```python
from build123d import *

# Parameters (mm, degrees)
PAD_DEPTH       = 15
FILLET_R        = 3
FILLET001_R     = 15
SKETCH001_R     = 2.75
POCKET_DEPTH    = 5.001
SKETCH002_R     = 5.1
PAD001_DEPTH    = 3
SKETCH003_R     = 4.1
POCKET001_DEPTH = 28.001
FILLET002_R     = 4


with BuildPart() as part:
    # Sketch → Pad (new body)
    with BuildSketch(Plane.XY):
        Polygon((0, 0), (0, 83), (5, 83), (5, 73), (25, 73), (25, 48), (135, 48), (135, 40), (5, 40), (5, 0), align=None)
    extrude(amount=PAD_DEPTH)

    # Fillet
    fillet_edges = [part.edges().sort_by_distance(p)[0] for p in [
        (25, 48, 7.5),
    ]]
    fillet(fillet_edges, radius=FILLET_R)

    # Fillet001
    fillet001_edges = [part.edges().sort_by_distance(p)[0] for p in [
        (5, 40, 7.5),
    ]]
    fillet(fillet001_edges, radius=FILLET001_R)

    # Sketch001 → Pocket (cut, through all)
    with BuildSketch(Plane.YZ.offset(5)):
        with Locations((7.5, 7.5)):
            Circle(SKETCH001_R)
        with Locations((78, 7.5)):
            Circle(SKETCH001_R)
    extrude(amount=-POCKET_DEPTH, mode=Mode.SUBTRACT)

    # Sketch002 → Pad001 (new body)
    with BuildSketch(Plane.YZ.offset(25)):
        with Locations((68, 7.5)):
            Circle(SKETCH002_R)
    extrude(amount=PAD001_DEPTH)

    # Sketch003 → Pocket001 (cut, through all)
    with BuildSketch(Plane.YZ.offset(28)):
        with Locations((68, 7.5)):
            Circle(SKETCH003_R)
    extrude(amount=-POCKET001_DEPTH, mode=Mode.SUBTRACT)

    # Fillet002
    fillet002_edges = [part.edges().sort_by_distance(p)[0] for p in [
        (77.5, 40, 15),
        (77.5, 40, 0),
    ]]
    fillet(fillet002_edges, radius=FILLET002_R)


solid = part.part
```
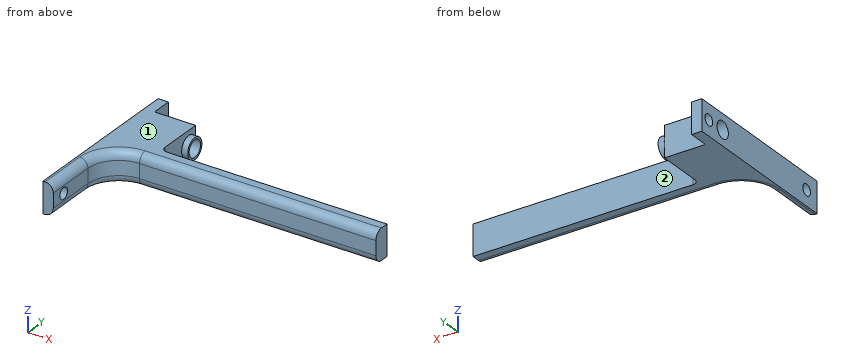
Verification items for the finished model (mm, model axes). Face numbers are marked on the shaded views. A direction names the side the tool comes from. Give positions to 0.01 mm unless a question says otherwise; leave off trailing zeros. Loops run counter-clockwise (first coordinate to the right, second up) from the corner with the lowest first, then second, coordinate; pieces in that order, holes last.
1. Section check A-A, the plane y = 7.5. Enter the section's corners in (x, z), then the cut area to 3 significant figures.
2. Set-up check for the marked faces 1 and 2: record each of +Z, -Z, +X, -X, +Y, -Y from which the full face is reachable in a straight line by a thin tool's end or side.
3. Section check C-C, the plane x = 112. Enter the section's corners in (y, z), then the cut area to 3 significant figures.
4. Section check B-B, the plane y = 78. Enter the section's corners in (x, z).
5. Section check D-D, the plane y = 68. Enter the section's corners in (x, z).
6. Thickness scan on line 1 (Z direction, x = 8, y = 68); line 2 (Z direction, x = 1.4, y = 7.5); line 3 (X direction, y = 24, z = 4). Record the ranges inside material, lowest first.
7. Go/stop test with flat-tipped pins: pin 1 Ø4 at (x, z) = (111, 7) entering from -Y; pin 2 Ø7.5 at (y, z) = (16.5, 8.5) entering from +X; pin 3 Ø7.5 at (x, z) = (17.5, 8.5) entering from +Y. Record where each tip stops, or that it passes through.
Geometry says:
1. outline: (0, 0) - (1, 0) arc R4 ccw to (5, 4) - (5, 4.75) - (0, 4.75) - close; (0, 10.25) - (5, 10.25) - (5, 11) arc R4 ccw to (1, 15) - (0, 15) - close
1. area: 40.6 mm2
2. face 1: +Z, +X, -X, +Y, -Y
2. face 2: +Z, -Z, +X, +Y
3. outline: (40, 4) arc R4 ccw to (44, 0) - (48, 0) - (48, 15) - (44, 15) arc R4 ccw to (40, 11) - close
3. area: 113 mm2
4. outline: (0, 0) - (5, 0) - (5, 4.75) - (0, 4.75) - close; (0, 10.25) - (5, 10.25) - (5, 15) - (0, 15) - close
5. outline: (0, 0) - (25, 0) - (25, 2.4) - (28, 2.4) - (28, 3.4) - (0, 3.4) - close; (0, 11.6) - (28, 11.6) - (28, 12.6) - (25, 12.6) - (25, 15) - (0, 15) - close
6. line 1: z = 0 to 3.4, 11.6 to 15
6. line 2: z = 0.02 to 4.75, 10.25 to 14.98
6. line 3: x = 0 to 5
7. pin 1: stops at y = 40
7. pin 2: stops at x = 5
7. pin 3: stops at y = 73
